Design review of the part built by this model. Coordinates are the model's own, in mm. A direction names the side the tool comes from. Round coordinates to 2 decimals unless told otherwise and drop trailing zeros. Order: outer loops, then holes, each group sorted by start corner. A loop starts at its lowest first (then second) coordinate and runs counter-clockwise, first axis right, second up. Notation, with made-up numbers: (66.25, 66.5) - (125.25, 66.5) arc R7 ccw to (125.25, 76.5) - close; hole circle Ø2 at (43.5, -27). An arc over 180 degrees is marked (long way). Answer as a JSON object with one key per item and string values. Group by question number.
from build123d import *

# Parameters (mm, degrees)
F1_DEPTH = 25.4
F3_DEPTH = 25.4


with BuildPart() as f1:
    # F0 (on Front) → F1 (new body)
    with BuildSketch(Plane.XZ):
        Polygon((27.711272, 14.598642), (-34.966588, 13.805252), (-34.966588, -38.392708), (27.711272, -38.392708), align=None)
        Polygon((-29.726638, -34.160443), (-31.742003, 9.774522), (22.471322, 9.169912), (21.04733, -33.517734), align=None, mode=Mode.SUBTRACT)
    extrude(amount=F1_DEPTH)

    # F2 (on Front) → F3 (join)
    with BuildSketch(Plane.XZ):
        Polygon((-21.46364, 37.788097), (-8.162229, 13.805252), (-4.937645, 13.805252), (-16.926625, 40.304425), align=None)
        Polygon((12.999105, 37.788097), (0, 13.805252), (4.736108, 13.805252), (18.642128, 37.788097), align=None)
    extrude(amount=F3_DEPTH)


solid = f1.part
1. To check wall thickness, follow line 1 (Z direction, x = 5.5, y = -6.5); line 2 (Z direction, x = 16.5, y = -17.5); line 3 (Z direction, x = -0.5, y = -11.25). State the ranges of each line that lie inside material, in increasing order. Write a range as from..to.
2. Tool access review of faces 1 (the flat face through (-10.935, -12.522, 27.061)), 2 (the flat face through (27.711, -13, -12)), 3 (the flat face through (-30.72, -12.52, -12.5)): name each direction out of +Z, -Z, +X, -X, +Y, -Y from which nothing blocks a thin tool from reaching the whole face with its end or side.
3. Mouldability with a two-part tool opening along Z and no side actions: class faces 4 (the flat face through (16, -13, 37.788)), 5 (the flat face through (-15, -12.52, 26.13)), 6 (the flat face through (11.741, -12.522, 25.885)), 7 (the flat face through (3, -25.4, 10)) as pulls with the +Z half, pulls with the -Z half, needs draft (parallel to the pull), parting line crosses it, or undercut.
4. Take a section at C-C, the plane y = -17.75. Give the boundary of the cut face in (x, z).
5. Clearance check with flat-ended pins moving along their axes: P1, Ø6, axis at x = 17, y = -15.5, coming from the +Z side; P2, Ø1.5, axis at x = 3.5, y = -15.5, coming from the +Z side. State where each tip first meets the part, or that it passes through.
6. Take a section at D-D, the plane x = 3. Give the boundary of the cut face in (y, z).
7. Take a section at B-B, the plane x = -18. Give the boundary of the cut face in (y, z).
8. Take a section at A-A, the plane z = -26. Give the boundary of the cut face in (x, y).
Response values:
{
 "1": {"line 1": "-38.39..-33.71, 9.36..14.32, 15.12..23.95", "line 2": "-38.39..-33.58, 9.24..14.46, 34.09..37.79", "line 3": "-38.39..-33.79, 9.43..14.24"},
 "2": {"face 1": "+Z, +Y, -Y", "face 2": "+Z, -Z, +X, +Y, -Y", "face 3": "+Y, -Y"},
 "3": {"face 4": "pulls with the +Z half", "face 5": "undercut", "face 6": "undercut", "face 7": "needs draft"},
 "4": {"outline": "(-34.97, -38.39) - (27.71, -38.39) - (27.71, 14.6) - (5.03, 14.31) - (18.64, 37.79) - (13, 37.79) - (0.24, 14.25) - (-5.11, 14.18) - (-16.93, 40.3) - (-21.46, 37.79) - (-8.35, 14.14) - (-34.97, 13.81) - close; hole (-31.74, 9.77) - (-29.73, -34.16) - (21.05, -33.52) - (22.47, 9.17) - close"},
 "5": {"P1": "z = 37.79", "P2": "z = 21.65"},
 "6": {"outline": "(-25.4, -38.39) - (0, -38.39) - (0, -33.75) - (-25.4, -33.75) - close; (-25.4, 9.39) - (0, 9.39) - (0, 19.34) - (-25.4, 19.34) - close"},
 "7": {"outline": "(-25.4, -38.39) - (0, -38.39) - (0, -34.01) - (-25.4, -34.01) - close; (-25.4, 9.62) - (0, 9.62) - (0, 14.02) - (-25.4, 14.02) - close; (-25.4, 31.54) - (0, 31.54) - (0, 39.71) - (-25.4, 39.71) - close"},
 "8": {"outline": "(-34.97, -25.4) - (-30.1, -25.4) - (-30.1, 0) - (-34.97, 0) - close; (21.3, -25.4) - (27.71, -25.4) - (27.71, 0) - (21.3, 0) - close"}
}
